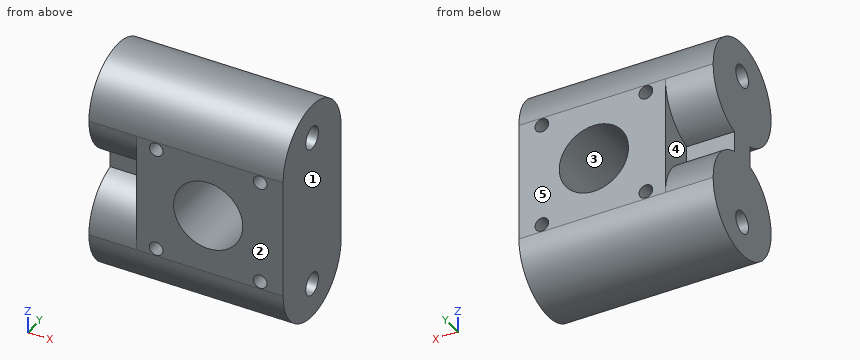
from build123d import *

# Parameters (mm, degrees)
SKETCH1_W             = 35
SKETCH1_H             = 32.5
BOSS_EXTRUDE1_DEPTH   = 15
SKETCH2_R             = 5.08
CUT_EXTRUDE2_DEPTH    = 30
SKETCH4_R             = 1
CUT_EXTRUDE3_DEPTH    = 15
M4X0_7_TAPPED_HOLE1_D = 3.3
FILLET1_RADIUS        = 7.5
FILLET1_LENGTH        = 35
FILLET2_RADIUS        = 7.5
FILLET2_LENGTH        = 35
SKETCH19_W            = 6.5
SKETCH19_H            = 32.5
CUT_EXTRUDE13_DEPTH   = 29.201285432
CUT_EXTRUDE14_START   = -7
CUT_EXTRUDE14_DEPTH   = 7


# Read off the part's stored shape, not the designer's step: Cut-Extrude14
with BuildPart() as part:
    # Sketch1 → Boss-Extrude1 (new body)
    with BuildSketch(Plane(origin=(0, 0, 0), x_dir=(1, 0, 0), z_dir=(0, 1, 0))):
        Rectangle(SKETCH1_W, SKETCH1_H)
    extrude(amount=-BOSS_EXTRUDE1_DEPTH)

    # Sketch2 → Cut-Extrude2 (cut)
    with BuildSketch(Plane(origin=(0, 0, 0), x_dir=(1, 0, 0), z_dir=(0, 1, 0))):
        with Locations(Location((0, 0, 0), (0, 0, 270))):
            Circle(SKETCH2_R)
    extrude(amount=-CUT_EXTRUDE2_DEPTH, mode=Mode.SUBTRACT)

    # Sketch4 → Cut-Extrude3 (cut)
    with BuildSketch(Plane(origin=(0, 0, 0), x_dir=(1, 0, 0), z_dir=(0, 1, 0))):
        with Locations(Location((7.633, 7.633, 0), (0, 0, 270))):
            Circle(SKETCH4_R)
        with Locations(Location((-7.633, 7.633, 0), (0, 0, 270))):
            Circle(SKETCH4_R)
        with Locations(Location((-7.633, -7.633, 0), (0, 0, 270))):
            Circle(SKETCH4_R)
        with Locations(Location((7.633, -7.633, 0), (0, 0, 270))):
            Circle(SKETCH4_R)
    extrude(amount=-CUT_EXTRUDE3_DEPTH, mode=Mode.SUBTRACT)

    # M4x0.7 Tapped Hole1 (through all)
    with Locations(Plane(origin=(-17.5, 0, 0), x_dir=(0, -1, 0), z_dir=(-1, 0, 0))):
        with Locations((7.5, -11.25), (7.5, 11.25)):
            Hole(M4X0_7_TAPPED_HOLE1_D / 2)

    # Fillet1: full round fillet: the end face becomes a half cylinder, R = half its width
    fillet1_face = Plane((0, -7.5, -16.25), x_dir=(1, 0, 0), z_dir=(0, 0, -1))  # on the end face: x along it, z out of the body
    fillet1_slab = fillet1_face.offset(-FILLET1_RADIUS / 2) * Box(FILLET1_LENGTH, 2 * FILLET1_RADIUS, FILLET1_RADIUS, mode=Mode.PRIVATE)  # the body's end, R deep
    fillet1_round = Plane((0, -7.5, -8.75), x_dir=(0, 0, -1), z_dir=(1, 0, 0)) * Cylinder(FILLET1_RADIUS, FILLET1_LENGTH, mode=Mode.PRIVATE)  # its axis R under the face
    add(fillet1_slab - fillet1_round, mode=Mode.SUBTRACT)

    # Fillet2: full round fillet: the end face becomes a half cylinder, R = half its width
    fillet2_face = Plane((0, -7.5, 16.25), x_dir=(1, 0, 0), z_dir=(0, 0, 1))  # on the end face: x along it, z out of the body
    fillet2_slab = fillet2_face.offset(-FILLET2_RADIUS / 2) * Box(FILLET2_LENGTH, 2 * FILLET2_RADIUS, FILLET2_RADIUS, mode=Mode.PRIVATE)  # the body's end, R deep
    fillet2_round = Plane((0, -7.5, 8.75), x_dir=(0, 0, 1), z_dir=(1, 0, 0)) * Cylinder(FILLET2_RADIUS, FILLET2_LENGTH, mode=Mode.PRIVATE)  # its axis R under the face
    add(fillet2_slab - fillet2_round, mode=Mode.SUBTRACT)

    # Sketch19 → Cut-Extrude13 (cut, through all)
    with BuildSketch(Plane.XZ.offset(15)):
        with Locations((14.25, 0)):
            Rectangle(SKETCH19_W, SKETCH19_H)
    extrude(amount=-CUT_EXTRUDE13_DEPTH, mode=Mode.SUBTRACT)

    # Cut-Extrude14 outline → Cut-Extrude14 (cut)
    with BuildSketch(Plane.ZY.offset(17.5).offset(CUT_EXTRUDE14_START)):
        with BuildLine():
            Line((-1.521583853, -5.5), (1.521583853, -5.5))
            ThreePointArc((1.521583853, -5.5), (4.208524469, -1.531331807), (8.75, 0))
            Line((8.75, 0), (-8.75, 0))
            ThreePointArc((-8.75, 0), (-4.208524469, -1.531331807), (-1.521583853, -5.5))
        make_face()
        with BuildLine():
            Line((-8.75, -15), (8.75, -15))
            ThreePointArc((8.75, -15), (4.208524469, -13.468668193), (1.521583853, -9.5))
            Line((1.521583853, -9.5), (-1.521583853, -9.5))
            ThreePointArc((-1.521583853, -9.5), (-4.208524469, -13.468668193), (-8.75, -15))
        make_face()
    extrude(amount=CUT_EXTRUDE14_DEPTH, mode=Mode.SUBTRACT)


solid = part.part
Geometry: final body of the model. Coordinates: model frame, mm. Face numbers are marked on the shaded views. A direction names the side the tool comes from. Give positions to 0.01 mm unless a question says otherwise; leave off trailing zeros. Loops run counter-clockwise (first coordinate to the right, second up) from the corner with the lowest first, then second, coordinate; pieces in that order, holes last. Notation, with made-up numbers: M -2,-24 L 7,-24 A18 ccw 7,-2 Z; hole C 49,-1 d4. An arc over 180 degrees is marked long. Put each result on its own line as item: value. Start each with the question number.
1) Cut plane C-C (x = 7). Output: boundary loops of the cut face in (y, z), then the cut area to 3 significant figures.
2) Pull-direction query (X, two-part tool) for the marked faces 1, 2 and 3; classes: pulls with the +X half, pulls with the -X half, needs draft (parallel to the pull), parting line crosses it, or undercut.
3) Contact query for flat-ended pins moving along their axis: pin 1 (6 mm diameter, centred on x = -1, y = -3.5, fed in from -Z); pin 2 (0.9 mm diameter, centred on x = -13, z = -0.5, fed in from +Y); pin 3 (3.5 mm diameter, centred on x = -13, z = -0.5, fed in from -Y). Output: stop coordinate, or through.
4) Access query for the marked faces 4 and 5. Directions: +Z, -Z, +X, -X, +Y, -Y. A direction counts if a zero-diameter tool reaches every point of the face in a straight line with its end or side. Return the directions, or none.
5) Cut plane B-B (z = 0). Output: boundary loops of the cut face in (x, y).
6) Ray query, line 1 along Z through (x, y) = (-8, -4); line 2 along Z through (x, y) = (-8.5, -11); line 3 along Z through (x, y) = (7.75, -6.25). Return the intervals inside material, ascending.
7) Cut plane A-A (x = 0). Output: boundary loops of the cut face in (y, z).
8) Cut plane D-D (y = -10). Output: boundary loops of the cut face in (x, z), then the cut area to 3 significant figures.
Verdict:
1. outline: M -15,-8.75 A7.5 ccw 0,-8.75 L 0,-8.41 L -15,-8.41 Z; M -15,-6.86 L 0,-6.86 L 0,6.86 L -15,6.86 Z; M -15,8.41 L 0,8.41 L 0,8.75 A7.5 ccw -15,8.75 Z; hole C -7.5,-11.25 d3.3; hole C -7.5,11.25 d3.3
1. area: 376 mm2
2. face 1: pulls with the +X half
2. face 2: needs draft
2. face 3: undercut
3. pin 1: z = -16.18
3. pin 2: y = -5.5
3. pin 3: y = -11.24
4. face 4: -X, +Y
4. face 5: +Z, -Z, +X, -X, +Y
5. outline: M -17.5,-9.5 L -10.5,-9.5 L -10.5,-15 L -5.08,-15 L -5.08,0 L -10.5,0 L -10.5,-5.5 L -17.5,-5.5 Z; M 5.08,-15 L 11,-15 L 11,0 L 5.08,0 Z
6. line 1: -15.38 to -8.56, -6.7 to 6.7, 8.56 to 15.38
6. line 2: -15.38 to -8.13, -7.13 to 7.13, 8.13 to 15.38
6. line 3: -16.15 to -12.33, -10.17 to -8.63, -6.64 to 6.64, 8.63 to 10.17, 12.33 to 16.15
7. outline: M -15,-8.75 A7.5 ccw 0,-8.75 L 0,-5.08 L -15,-5.08 Z; M -15,5.08 L 0,5.08 L 0,8.75 A7.5 ccw -15,8.75 Z; hole C -7.5,-11.25 d3.3; hole C -7.5,11.25 d3.3
8. outline: M -17.5,-15.82 L 11,-15.82 L 11,15.82 L -17.5,15.82 L -17.5,1.68 L -10.5,1.68 L -10.5,-1.68 L -17.5,-1.68 Z; hole C -7.63,-7.63 d2; hole C -7.63,7.63 d2; hole C 0,0 d10.16; hole C 7.63,-7.63 d2; hole C 7.63,7.63 d2
8. area: 785 mm2
